For this review, take the finished solid that the model builds, in its own axes (mm). Face numbers are marked on the shaded views. A direction names the side the tool comes from. Round coordinates to 2 decimals unless told otherwise and drop trailing zeros. Order: outer loops, then holes, each group sorted by start corner. A loop starts at its lowest first (then second) coordinate and runs counter-clockwise, first axis right, second up. Notation, with made-up numbers: (-15, 71.25) - (18, 71.25) arc R6 cw to (18, 80.25) - close; hole circle Ø1 at (33.25, 24.5). An arc over 180 degrees is marked (long way). One line per question, with ' | ' between items.
```python
from build123d import *

# Parameters (mm, degrees)
F0_R     = 12.7
F0_R_2   = 7.9375
F1_DEPTH = 6.35
F0_R_3   = 4.7625
F2_DEPTH = 24.60625
F3_R     = 4.7625
F3_R_2   = 3.175
F4_DEPTH = 5.08
F5_DEPTH = 5.08
F6_D     = 5.4102


with BuildPart() as f1:
    # F0 (on Right) → F1 (new body)
    with BuildSketch(Plane.YZ):
        Circle(F0_R)
        Circle(F0_R_2, mode=Mode.SUBTRACT)
    extrude(amount=F1_DEPTH)

    # F0 (on Right) → F2 (join)
    with BuildSketch(Plane.YZ):
        Circle(F0_R_2)
        Circle(F0_R_3, mode=Mode.SUBTRACT)
    extrude(amount=F2_DEPTH)

    # F3 (on face) → F4 (join)
    with BuildSketch(Plane.YZ.offset(24.60625)):
        Circle(F3_R)
        Circle(F3_R_2, mode=Mode.SUBTRACT)
    extrude(amount=-F4_DEPTH)

    # F3 (on face) → F5 (join)
    with BuildSketch(Plane.YZ.offset(24.60625)):
        Circle(F3_R_2)
    extrude(amount=-F5_DEPTH)

    # F6 (through all)
    with Locations(Plane.YZ.offset(24.60625)):
        with Locations((0, 0)):
            Hole(F6_D / 2)


solid = f1.part
```
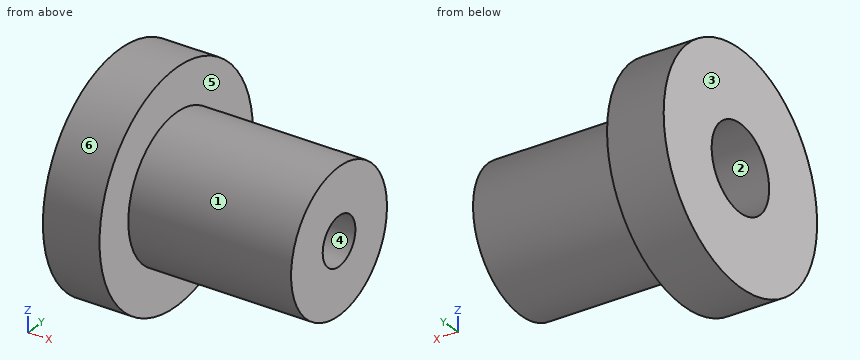
(1) For probe 1 along Z at (x, y) = (8.5, 0); probe 2 along Z at (x, y) = (22.65, 0); probe 3 along X at (y, z) = (-10, -1.5), list the stretches that pass through material, from the lowest coordinate up. Write a range as [from, to].
Output values:
probe 1: [-7.94, -4.76], [4.76, 7.94] | probe 2: [-7.94, -2.71], [2.71, 7.94] | probe 3: [0, 6.35]
(2) We need section C-C on x = 20. State the section outline as (y, z) points (1 decimal).
Output values:
outline: circle Ø15.9 at (0, 0); hole circle Ø5.4 at (0, 0)
(3) Mouldability with a two-part tool opening along Y and no side actions: class the marked faces 1, 2, 3 and 4 as released by +Y, released by -Y, zero draft, split by the parting line, or undercut.
Output values:
face 1: split by the parting line | face 2: undercut | face 3: zero draft | face 4: undercut
(4) For the marked faces 5 and 6, list the 3-axis set-ups (+Z, -Z, +X, -X, +Y, -Y) from which the entire face can be reached by the end or side of a thin tool; tool diameter is ignored.
Output values:
face 5: +X | face 6: +X, -X
(5) We need section A-A on z = 0. State the section outline as (x, y) points, plus the area to 3 significant figures.
Output values:
outline: (0, -12.7) - (6.35, -12.7) - (6.35, -7.94) - (24.61, -7.94) - (24.61, -2.71) - (19.53, -2.71) - (19.53, -4.76) - (0, -4.76) - close; (0, 4.76) - (19.53, 4.76) - (19.53, 2.71) - (24.61, 2.71) - (24.61, 7.94) - (6.35, 7.94) - (6.35, 12.7) - (0, 12.7) - close | area: 238 mm^2
(6) We need section D-D on z = -6.25. State the section outline as (x, y) points.
Output values:
outline: (0, -11.06) - (6.35, -11.06) - (6.35, -4.89) - (24.61, -4.89) - (24.61, 4.89) - (6.35, 4.89) - (6.35, 11.06) - (0, 11.06) - close
(7) Insertion check: pin 1 (5 mm diameter, centred on x = 21, y = 9, fed in from +Z); pin 2 (6 mm diameter, centred on x = 21, y = -6, fed in from +Z); pin 3 (12.5 mm diameter, centred on y = 0, z = 0, fed in from +X); pin 4 (1.5 mm diameter, centred on x = 6.5, z = -7.5, fed in from +Y). Each pin has a flat end and moves straight along its axis. Give the tip position at first contact, or say it passes through.
Output values:
pin 1: z = 4.56 | pin 2: z = 7.35 | pin 3: x = 24.61 | pin 4: y = 10.75
